Here's the drawing with two shaded views (mm, measured from the low corner). I have some questions. A direction names the side the tool comes from. Give positions to 0.01 mm unless a question says otherwise; leave off trailing zeros. Loops run counter-clockwise (first coordinate to the right, second up) from the corner with the lowest first, then second, coordinate; pieces in that order, holes last. Notation, with made-up numbers: M 57,26 L 108,26 A21 cw 108,52 Z; hole C 63,-32.75 d9. An arc over 180 degrees is marked long. Use a Markdown table: item, result. Add a question column.
1) Which directions (+Z, -Z, +X, -X, +Y, -Y) give clear straight access to the entire face, cutting with the end or side of a thin tool? Please do the marked faces 5 and 6.
2) Suppose I cut it at A-A on z = 6. List the corners of the cut face in (x, y) for me (1 decimal), and give its area (3 significant figures).
3) Suppose I cut it at D-D on y = 38.5. List the corners of the cut face in (x, z) for me, and give its area (3 significant figures).
4) If I drill on line 1 along Y through (x, z) = (3.5, 0.4); line 2 along X through (y, z) = (36.5, 2.5); line 3 along Z through (x, y) = (110, 4), over which ranges is the centre line in solid material (lowest first)? Write a range as [from, to].
5) Suppose I cut it at C-C on y = 3.5. List the corners of the cut face in (x, z) for me, and give its area (3 significant figures).
6) Will these pins go through, and if not, where does the flat tip stop? pin 1 Ø1 at (y, z) = (31, 13.5) entering from +X; pin 2 Ø2 at (y, z) = (27, 3.5) entering from -X; pin 3 Ø5 at (x, z) = (115, 11) entering from +Y.
7) We'd pull the mould along X, two halves only. Please class the marked faces 1, 2, 3 and 4: +X half, -X half, draft (parallel to the pull), parting line (faces both ways), or undercut.
8) Suppose I cut it at B-B on x = 116.5. List the corners of the cut face in (y, z) for me (1 decimal).
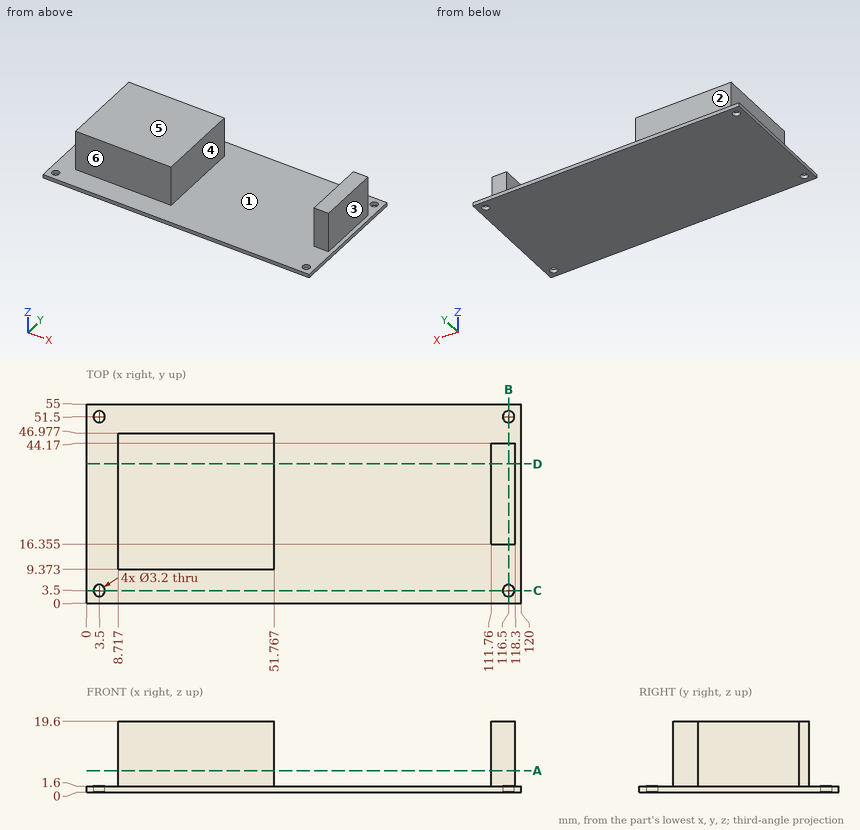
Answer block:
| question | item | result |
|---|---|---|
| 1 | face 5 | +Z, +X, -X, +Y, -Y |
| 1 | face 6 | +Z, +X, -X, -Y |
| 2 | outline | M 8.7,9.4 L 51.8,9.4 L 51.8,47 L 8.7,47 Z; M 111.8,16.4 L 118.3,16.4 L 118.3,44.2 L 111.8,44.2 Z |
| 2 | area | 1,800 mm^2 |
| 3 | outline | M 0,0 L 120,0 L 120,1.6 L 118.3,1.6 L 118.3,19.6 L 111.76,19.6 L 111.76,1.6 L 51.77,1.6 L 51.77,19.6 L 8.72,19.6 L 8.72,1.6 L 0,1.6 Z |
| 3 | area | 1,080 mm^2 |
| 4 | line 1 | y = [0, 1.9], [5.1, 49.9], [53.1, 55] |
| 4 | line 2 | x = [8.72, 51.77], [111.76, 118.3] |
| 4 | line 3 | z = [0, 1.6] |
| 5 | outline | M 0,0 L 1.9,0 L 1.9,1.6 L 0,1.6 Z; M 5.1,0 L 114.9,0 L 114.9,1.6 L 5.1,1.6 Z; M 118.1,0 L 120,0 L 120,1.6 L 118.1,1.6 Z |
| 5 | area | 182 mm^2 |
| 6 | pin 1 | stops at x = 118.3 |
| 6 | pin 2 | stops at x = 8.72 |
| 6 | pin 3 | stops at y = 44.17 |
| 7 | face 1 | undercut |
| 7 | face 2 | draft |
| 7 | face 3 | +X half |
| 7 | face 4 | undercut |
| 8 | outline | M 0,0 L 1.9,0 L 1.9,1.6 L 0,1.6 Z; M 5.1,0 L 49.9,0 L 49.9,1.6 L 44.2,1.6 L 44.2,19.6 L 16.4,19.6 L 16.4,1.6 L 5.1,1.6 Z; M 53.1,0 L 55,0 L 55,1.6 L 53.1,1.6 Z |
